```python
from build123d import *

# Parameters (mm, degrees)
F1_DEPTH  = 85
F2_R      = 2
F3_DEPTH  = 10
F4_W      = 19.472218
F4_H      = 61.057516
F4_W_2    = 18.561906
F5_DEPTH  = 25
F8_DEPTH  = 50
F10_DEPTH = 30
F11_W     = 10.871612
F11_H     = 24.349149
F12_DEPTH = 5
F13_R     = 1
F14_DEPTH = 7


with BuildPart() as f1:
    # F0 (on Top) → F1 (new body)
    with BuildSketch(Plane.XY):
        Polygon((15, 42.5), (-15, 42.5), (-15, 15.500662), (-10.938493, 15.500662), (-10.938493, -15.873631), (-15, -15.873631), (-15, -42.5), (15, -42.5), align=None)
    extrude(amount=F1_DEPTH)

    # F2 (on face) → F3 (cut)
    with BuildSketch(Plane.YZ.offset(15)):
        with Locations((-37.5, 5)):
            Circle(F2_R)
        with Locations((37.5, 5)):
            Circle(F2_R)
        with Locations((37.5, 80)):
            Circle(F2_R)
        with Locations((-37.5, 80)):
            Circle(F2_R)
    extrude(amount=-F3_DEPTH, mode=Mode.SUBTRACT)

    # F4 (on face) → F5 (cut)
    with BuildSketch(Plane.YZ.offset(15)):
        with Locations((-42.5, 42.5)):
            Rectangle(F4_W, F4_H)
        with Locations((42.5, 42.5)):
            Rectangle(F4_W_2, F4_H)
    extrude(amount=-F5_DEPTH, mode=Mode.SUBTRACT)

    # F7 (on offset) → F8 (join)
    with BuildSketch(Plane.XY.offset(15)):
        Polygon((-4.637186, 48.255824), (-4.637186, 33.027273), (2.820976, 33.027273), (2.820976, 41.918974), (9.94103, 41.918974), (9.94103, 48.255824), (2.820976, 48.255824), align=None)
    extrude(amount=F8_DEPTH)

    # F9 (on offset) → F10 (join)
    with BuildSketch(Plane.XY.offset(15)):
        Polygon((2.636472, -32.500222), (-4.438653, -32.500222), (-4.438653, -49.462382), (2.636472, -49.462382), (10.165131, -49.462382), (10.165131, -41.752309), (2.636472, -41.752309), align=None)
    extrude(amount=F10_DEPTH)

    # F11 (on face) → F12 (join)
    with BuildSketch(Plane.YZ.offset(-10)):
        with Locations((-39.88678, 58.680521)):
            Rectangle(F11_W, F11_H)
    extrude(amount=F12_DEPTH)

    # F13 (on face) → F14 (join)
    with BuildSketch(Plane.YZ.offset(-5)):
        with BuildLine():
            Line((-36.450974, 52.248876), (-36.450974, 64.410565))
            ThreePointArc((-36.450974, 64.410565), (-36.881787, 65.232773), (-37.803027, 65.346545))
            Line((-37.803027, 65.346545), (-42.803027, 63.465884))
            ThreePointArc((-42.803027, 63.465884), (-43.273182, 63.099091), (-43.450974, 62.529904))
            Line((-43.450974, 62.529904), (-43.450974, 53.939643))
            ThreePointArc((-43.450974, 53.939643), (-43.263481, 53.356691), (-42.771309, 52.992339))
            Line((-42.771309, 52.992339), (-37.771309, 51.301572))
            ThreePointArc((-37.771309, 51.301572), (-36.868022, 51.436369), (-36.450974, 52.248876))
        make_face()
        Polygon((-42.087062, 68.266637), (-40.955583, 66.253409), (-38.646336, 66.226684), (-37.468569, 68.213188), (-38.600048, 70.226416), (-40.909294, 70.253141), align=None)
        with Locations((-39.777815, 68.239912)):
            Circle(F13_R, mode=Mode.SUBTRACT)
        Polygon((-42.087215, 49.099645), (-40.929939, 47.101134), (-38.62054, 47.104108), (-37.468416, 49.105594), (-38.625692, 51.104105), (-40.935091, 51.10113), align=None)
        with Locations((-39.777815, 49.102619)):
            Circle(F13_R, mode=Mode.SUBTRACT)
    extrude(amount=F14_DEPTH)


solid = f1.part
```
The model under review builds one solid part; all positions refer to its coordinate system, in mm. A direction names the side the tool comes from. Give positions to 0.01 mm unless a question says otherwise; leave off trailing zeros. Order: outer loops, then holes, each group sorted by start corner. A loop starts at its lowest first (then second) coordinate and runs counter-clockwise, first axis right, second up. Notation, with made-up numbers: (50.25, 18) - (89.25, 18) arc R18 ccw to (89.25, 46) - close; hole circle Ø8 at (-40, 30.25). An arc over 180 degrees is marked (long way). Use CSV: the item, a comma, the result in double quotes. Start each with the question number.
Q1. We need section B-B, the plane x = -7. Write out the cut boundary in (y, z).
Q2. We need section D-D, the plane z = 76.5. Write out the cut boundary in (x, y), and give its area (3 significant figures).
Q3. Tool access review of faces 1 (the flat face through (-13, -15.874, 42)), 2 (the flat face through (-10.2, -42.5, 41.9)), 3 (the flat face through (-8, -40, 46.506)), 4 (the flat face through (5, 37, 80)): name each direction out of +Z, -Z, +X, -X, +Y, -Y from which nothing blocks a thin tool from reaching the whole face with its end or side.
Q4. We need section C-C, the plane z = 5. Write out the cut boundary in (x, y), and give its area (3 significant figures).
Q5. We need section A-A, the plane y = 37.5. Write out the cut boundary in (x, z).
Q6. To check wall thickness, follow line 1 along Z through (x, y) = (8.75, 37.5); line 2 along Y through (x, z) = (-11.5, 9.5); line 3 along Y through (x, z) = (6.5, 63.5). State the ranges of each line that lie inside material, in increasing order. Write a range as [from, to].
Q7. Clearance check with flat-ended pins moving along their axes: pin 1 Ø2 at (x, z) = (-0.5, 59.5) entering from -Y; pin 2 Ø6 at (y, z) = (-46, 31.5) entering from +X; pin 3 Ø5 at (y, z) = (-35.5, 39) entering from +X. State where each tip first meets the part, or that it passes through.
Q8. The part is to be moulded in two halves that separate along Y. For faces 5 (the flat face through (-2, -43.451, 58)), 6 (the flat face through (-4.439, -41, 30)), 7 (the cylindrical face through (-1.549, -38.854, 48.72)), say which applies: +Y half, -Y half, draft (parallel to the pull), parting line (faces both ways), or undercut.
Outcome:
1,outline,"(-45.32, 46.51) - (-34.45, 46.51) - (-34.45, 70.86) - (-45.32, 70.86) - close; (-42.5, 0) - (42.5, 0) - (42.5, 11.97) - (33.22, 11.97) - (33.22, 73.03) - (42.5, 73.03) - (42.5, 85) - (-42.5, 85) - (-42.5, 73.03) - (-32.76, 73.03) - (-32.76, 11.97) - (-42.5, 11.97) - close"
2,outline,"(-15, -42.5) - (15, -42.5) - (15, 42.5) - (-15, 42.5) - (-15, 15.5) - (-10.94, 15.5) - (-10.94, -15.87) - (-15, -15.87) - close"
2,area,"2,420 mm^2"
3,face 1,"+Z, -Z, -X"
3,face 2,"-X, -Y"
3,face 3,"+X, -Y"
3,face 4,"+X"
4,outline,"(-15, -42.5) - (15, -42.5) - (15, -39.5) - (5, -39.5) - (5, -35.5) - (15, -35.5) - (15, 35.5) - (5, 35.5) - (5, 39.5) - (15, 39.5) - (15, 42.5) - (-15, 42.5) - (-15, 15.5) - (-10.94, 15.5) - (-10.94, -15.87) - (-15, -15.87) - close"
4,area,"2,340 mm^2"
5,outline,"(-15, 0) - (15, 0) - (15, 3) - (5, 3) - (5, 7) - (15, 7) - (15, 11.97) - (-10, 11.97) - (-10, 73.03) - (15, 73.03) - (15, 78) - (5, 78) - (5, 82) - (15, 82) - (15, 85) - (-15, 85) - close; (-4.64, 15) - (2.82, 15) - (2.82, 65) - (-4.64, 65) - close"
6,line 1,"z = [0, 3], [7, 11.97], [73.03, 78], [82, 85]"
6,line 2,"y = [-42.5, -15.87], [15.5, 42.5]"
6,line 3,"y = [-32.76, 33.22], [41.92, 48.26]"
7,pin 1,"stops at y = -43.45"
7,pin 2,"stops at x = 10.17"
7,pin 3,"stops at x = 2.64"
8,face 5,"-Y half"
8,face 6,"draft"
8,face 7,"undercut"
